Geometry check sheet. Reference: the model listing, model coordinates, mm. Face numbers are marked on the shaded views. A direction names the side the tool comes from. Coordinates: 2 decimals unless noted, no trailing zeros. Write each loop counter-clockwise with the first axis right and the second up, starting at its lowest first coordinate (ties: lowest second). Pieces come first, ordered by that corner, then holes. Notation, with made-up numbers: (17.25, -32.75) -> (76.25, -32.75) arc R13 ccw to (76.25, -25.75) -> close; hole circle Ø4 at (12, 85). An arc over 180 degrees is marked (long way). Answer in a Markdown table with one row per item. Add a question column.
Q1. Thickness scan on line 1 (X direction, y = -17.5, z = 1.4); line 2 (X direction, y = -17.5, z = 1.5); line 3 (Z direction, x = -27, y = -9.25). Record the ranges inside material, lowest first.
Q2. Section check C-C, the plane x = -47.5. Record the boundary of the cut face in (y, z).
Q3. Section check A-A, the plane z = 1.4. Record the boundary of the cut face in (x, y) (3 decimals).
Q4. Section check D-D, the plane y = -15.5. Count the separate pieces of the cut face and the enclosed holes in it, and give its area (3 significant figures).
Q5. Gauge pin test, flat ends, axial feed: P1, Ø4.5, axis at x = -41, y = -14.5, coming from the +Z side; P2, Ø5, axis at x = -51, y = -12.5, coming from the +Z side; P3, Ø6, axis at x = -60.5, y = -15, coming from the +Z side. Record the tip position at first contact, or that the pin passes through.
Q6. Release check for a two-part mould opening along X. For the marked faces 1, 2 and 3 record: pulls with the +X half, pulls with the -X half, needs draft (parallel to the pull), parting line crosses it, or undercut.
Q7. Tool access check on the marked faces 4 and 5. Record the directions out of +Z, -Z, +X, -X, +Y, -Y that give a thin tool (end or side, any length) a straight path to the whole face; none if there is none.
Q8. Section check B-B, the plane z = -0.5. Record the boundary of the cut face in (x, y) (3 decimals).
```python
from build123d import *

# Parameters (mm, degrees)
F0_R     = 4.3
F1_DEPTH = 2
F2_D     = 2.85
F2_DEPTH = 11
F2_TIP   = 0.8562263821
F3_DEPTH = 2.5
F5_SIZE  = 0.5


# Not quite as in the source:
# - a fillet or chamfer that OpenCascade refuses, or shapes differently, is made with other operations: its cross-section is extruded or revolved along the edge and cut away or added


with BuildPart() as f1:
    # F0 (on Top) → F1 (new body)
    with BuildSketch(Plane.XY):
        Polygon((-24.6178394498, -8.8684120262), (-63.6178394498, -8.8684120262), (-63.6178394498, -16.3684120262), (-63.6178394498, -23.8684120262), (-24.6178394498, -23.8684120262), (-24.6178394498, -16.3684120262), align=None)
        with BuildLine():
            ThreePointArc((-55.0178394498, -16.3684120262), (-59.3178394498, -20.6684120262), (-63.6178394498, -16.3684120262))
            ThreePointArc((-63.6178394498, -16.3684120262), (-59.3178394498, -12.0684120262), (-55.0178394498, -16.3684120262))
        make_face(mode=Mode.SUBTRACT)
        with Locations((-28.9178394498, -16.3684120262)):
            Circle(F0_R, mode=Mode.SUBTRACT)
        with BuildLine():
            ThreePointArc((-55.0178394498, -16.3684120262), (-59.3178394498, -12.0684120262), (-63.6178394498, -16.3684120262))
            ThreePointArc((-63.6178394498, -16.3684120262), (-59.3178394498, -20.6684120262), (-55.0178394498, -16.3684120262))
        make_face()
        Polygon((-59.3178394498, -13.1352505188), (-56.5178394498, -14.7518312725), (-56.5178394498, -17.98499278), (-59.3178394498, -19.6015735337), (-62.1178394498, -17.98499278), (-62.1178394498, -14.7518312725), align=None, mode=Mode.SUBTRACT)
        with Locations((-28.9178394498, -16.3684120262)):
            Circle(F0_R)
        Polygon((-28.9178394498, -13.1352505188), (-26.1178394498, -14.7518312725), (-26.1178394498, -17.98499278), (-28.9178394498, -19.6015735337), (-31.7178394498, -17.98499278), (-31.7178394498, -14.7518312725), align=None, mode=Mode.SUBTRACT)
        Polygon((-56.5178394498, -17.98499278), (-56.5178394498, -14.7518312725), (-59.3178394498, -13.1352505188), (-62.1178394498, -14.7518312725), (-62.1178394498, -17.98499278), (-59.3178394498, -19.6015735337), align=None)
        Polygon((-26.1178394498, -17.98499278), (-26.1178394498, -14.7518312725), (-28.9178394498, -13.1352505188), (-31.7178394498, -14.7518312725), (-31.7178394498, -17.98499278), (-28.9178394498, -19.6015735337), align=None)
    extrude(amount=-F1_DEPTH)

    # F2
    with Locations(Plane.XY):
        with Locations((-59.3178394498, -16.3684120262), (-28.9178394498, -16.3684120262)):
            Hole(F2_D / 2, depth=F2_DEPTH)
            with Locations((0, 0, -(F2_DEPTH + F2_TIP / 2))):  # 118° drill point
                Cone(0, F2_D / 2, F2_TIP, mode=Mode.SUBTRACT)

    # F0 (on Top) → F3 (join)
    with BuildSketch(Plane.XY):
        with BuildLine():
            ThreePointArc((-55.0178394498, -16.3684120262), (-59.3178394498, -12.0684120262), (-63.6178394498, -16.3684120262))
            ThreePointArc((-63.6178394498, -16.3684120262), (-59.3178394498, -20.6684120262), (-55.0178394498, -16.3684120262))
        make_face()
        Polygon((-59.3178394498, -13.1352505188), (-56.5178394498, -14.7518312725), (-56.5178394498, -17.98499278), (-59.3178394498, -19.6015735337), (-62.1178394498, -17.98499278), (-62.1178394498, -14.7518312725), align=None, mode=Mode.SUBTRACT)
        with Locations((-28.9178394498, -16.3684120262)):
            Circle(F0_R)
        Polygon((-28.9178394498, -13.1352505188), (-26.1178394498, -14.7518312725), (-26.1178394498, -17.98499278), (-28.9178394498, -19.6015735337), (-31.7178394498, -17.98499278), (-31.7178394498, -14.7518312725), align=None, mode=Mode.SUBTRACT)
    extrude(amount=F3_DEPTH)

    # F4: chamfer of 2.5 on 2 edges, made by hand


with BuildPart() as f4_tool2:
    # F4_s3 → F4_t4 (revolve)
    with BuildSketch(Plane.XZ.offset(16.3684120262)):
        Polygon((-66.1178394498, 0), (-63.6178394498, 2.5), (-63.6178394498, 0), align=None)
    revolve(axis=Axis((-59.3178394498, -16.3684120262, 0), (0, 0, 1)))

    split(bisect_by=Plane.YZ.offset(-63.6178394498), keep=Keep.TOP)


with BuildPart() as f1_1:
    add(f1.part)

    # F4_t1: union F4_tool2
    add(f4_tool2.part)


with BuildPart() as f4_tool7:
    # F4_s8 → F4_t9 (revolve)
    with BuildSketch(Plane.XZ.offset(16.3684120262)):
        Polygon((-22.1178394498, 0), (-24.6178394498, 2.5), (-24.6178394498, 0), align=None)
    revolve(axis=Axis((-28.9178394498, -16.3684120262, 0), (0, 0, 1)))

    split(bisect_by=Plane.YZ.offset(-24.6178394498), keep=Keep.BOTTOM)


with BuildPart() as f1_2:
    add(f1_1.part)

    # F4_t6: union F4_tool7
    add(f4_tool7.part)

    # F5
    f5_edges = [f1_2.edges().sort_by_distance(p)[0] for p in [
        (-63.617839, -16.368412, -2),
    ]]
    chamfer(f5_edges, length=F5_SIZE)


solid = f1_2.part
```
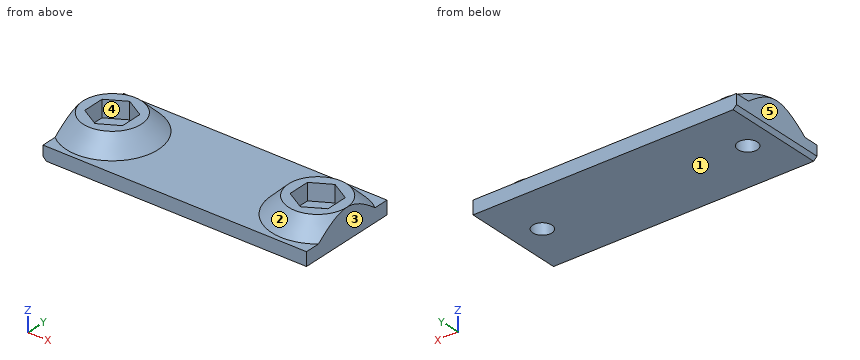
Calculated:
| question | item | result |
|---|---|---|
| 1 | line 1 | x = -63.62 to -62.12, -56.52 to -54.04, -34.2 to -31.72, -26.12 to -24.62 |
| 1 | line 2 | x = -63.62 to -62.12, -56.52 to -54.14, -34.1 to -31.72, -26.12 to -24.62 |
| 1 | line 3 | z = -2 to 0 |
| 2 | outline | (-23.87, -2) -> (-8.87, -2) -> (-8.87, 0) -> (-23.87, 0) -> close |
| 3 | outline | (-63.618, -19.635) arc R5.4 ccw (long way) to (-63.618, -13.102) -> close; (-24.618, -19.635) -> (-24.618, -13.102) arc R5.4 ccw (long way) to start; hole (-62.118, -17.985) -> (-59.318, -19.602) -> (-56.518, -17.985) -> (-56.518, -14.752) -> (-59.318, -13.135) -> (-62.118, -14.752) -> close; hole (-31.718, -17.985) -> (-28.918, -19.602) -> (-26.118, -17.985) -> (-26.118, -14.752) -> (-28.918, -13.135) -> (-31.718, -14.752) -> close |
| 4 | separate pieces | 3 |
| 4 | enclosed holes | 0 |
| 4 | area | 89.7 mm² |
| 5 | P1 | stops at z = 0 |
| 5 | P2 | stops at z = 0.13 |
| 5 | P3 | stops at z = 2.5 |
| 6 | face 1 | needs draft |
| 6 | face 2 | undercut |
| 6 | face 3 | pulls with the +X half |
| 7 | face 4 | +Z |
| 7 | face 5 | +Z, -Z, -X, +Y, -Y |
| 8 | outline | (-63.618, -23.868) -> (-24.618, -23.868) -> (-24.618, -8.868) -> (-63.618, -8.868) -> close; hole circle Ø2.85 at (-59.318, -16.368); hole circle Ø2.85 at (-28.918, -16.368) |
